Design review of the part built by this model. Coordinates are the model's own, in mm. A direction names the side the tool comes from. Coordinates: 2 decimals unless noted, no trailing zeros. Write each loop counter-clockwise with the first axis right and the second up, starting at its lowest first coordinate (ties: lowest second). Pieces come first, ordered by that corner, then holes. Notation, with made-up numbers: (61, 10) - (119, 10) arc R13 ccw to (119, 26) - close; hole circle Ø2 at (5.25, 66). An arc over 180 degrees is marked (long way). Answer as a JSON object with one key per item and string values.
```python
from build123d import *

# Parameters (mm, degrees)
SKETCH1_R           = 19.05
BOSS_EXTRUDE1_DEPTH = 31.75
SKETCH3_R           = 6.35
CUT_EXTRUDE1_DEPTH  = 127.593613969


with BuildPart() as part:
    # Sketch1 → Boss-Extrude1 (new, symmetric)
    with BuildSketch(Plane.XY):
        with BuildLine():
            Line((-51.074053478, -18.968891898), (-51.074053478, -6.268891898))
            ThreePointArc((-51.074053478, -6.268891898), (-54.793797356, 2.711364223), (-63.774053478, 6.431108102))
            Line((-63.774053478, 6.431108102), (-106.700053478, 6.431108102))
            Line((-106.700053478, 6.431108102), (-106.700053478, 14.381308102))
            Line((-106.700053478, 14.381308102), (58.399946522, 14.381308102))
            Line((58.399946522, 14.381308102), (58.399946522, 6.431108102))
            Line((58.399946522, 6.431108102), (15.473946522, 6.431108102))
            ThreePointArc((15.473946522, 6.431108102), (6.493690401, 2.711364223), (2.773946522, -6.268891898))
            Line((2.773946522, -6.268891898), (2.773946522, -18.968891898))
            ThreePointArc((2.773946522, -18.968891898), (-24.150053478, -45.892891898), (-51.074053478, -18.968891898))
        make_face()
        with Locations((-24.150053478, -18.968891898)):
            Circle(SKETCH1_R, mode=Mode.SUBTRACT)
    extrude(amount=BOSS_EXTRUDE1_DEPTH, both=True)

    # Sketch3 → Cut-Extrude1 (cut, through all)
    with BuildSketch(Plane(origin=(0, 14.381308102, 0), x_dir=(1, 0, 0), z_dir=(0, 1, 0))):
        with Locations(Location((-87.650053478, 15.875, 0), (0, 0, 270))):
            Circle(SKETCH3_R)
        with Locations(Location((-87.650053478, -15.875, 0), (0, 0, 270))):
            Circle(SKETCH3_R)
        with Locations(Location((39.349946522, -15.875, 0), (0, 0, 270))):
            Circle(SKETCH3_R)
        with Locations(Location((39.349946522, 15.875, 0), (0, 0, 270))):
            Circle(SKETCH3_R)
    extrude(amount=-CUT_EXTRUDE1_DEPTH, mode=Mode.SUBTRACT)


solid = part.part
```
(1) The part is to be moulded in two halves that separate along X. For faces 4 (the face through (-85, 6.431, 0)), 5 (the face through (-5.98, -13.25, -0.44)), 6 (the face through (-23.558, -45.886, 0.444)), say which applies: pulls with the +X half, pulls with the -X half, needs draft (parallel to the pull), parting line crosses it, or undercut.
Solved:
{"face 4": "needs draft", "face 5": "undercut", "face 6": "parting line crosses it"}
(2) Tool access review of faces 1 (the face through (2.774, -13, 0)), 2 (the face through (-81.354, 10.462, -16.702)), 3 (the face through (-51.074, -13, 0)): name each direction out of +Z, -Z, +X, -X, +Y, -Y from which nothing blocks a thin tool from reaching the whole face with its end or side.
Solved:
{"face 1": "+Z, -Z, +X, -Y", "face 2": "+Y, -Y", "face 3": "+Z, -Z, -X, -Y"}
(3) Take a section at D-D, the plane z = 17. Write out the cut boundary in (x, y), and give its area (3 significant figures).
Solved:
{"outline": "(-106.7, 6.43) - (-93.9, 6.43) - (-93.9, 14.38) - (-106.7, 14.38) - close; (-81.4, 6.43) - (-63.77, 6.43) arc R12.7 cw to (-51.07, -6.27) - (-51.07, -18.97) arc R26.92 ccw to (2.77, -18.97) - (2.77, -6.27) arc R12.7 cw to (15.47, 6.43) - (33.1, 6.43) - (33.1, 14.38) - (-81.4, 14.38) - close; (45.6, 6.43) - (58.4, 6.43) - (58.4, 14.38) - (45.6, 14.38) - close; hole circle Ø38.1 at (-24.15, -18.97)", "area": "2,550 mm^2"}
(4) Take a section at B-B, the plane x = -39. Write out the cut boundary in (y, z), and give its area (3 significant figures).
Solved:
{"outline": "(-41.43, -31.75) - (-30.9, -31.75) - (-30.9, 31.75) - (-41.43, 31.75) - close; (-7.04, -31.75) - (14.38, -31.75) - (14.38, 31.75) - (-7.04, 31.75) - close", "area": "2,030 mm^2"}
(5) Take a section at C-C, the plane y = -26.5. Write out the cut boundary in (x, z).
Solved:
{"outline": "(-50, -31.75) - (-41.65, -31.75) - (-41.65, 31.75) - (-50, 31.75) - close; (-6.65, -31.75) - (1.7, -31.75) - (1.7, 31.75) - (-6.65, 31.75) - close"}
(6) Take a section at A-A, the plane z = -8. Write out the cut boundary in (x, y), and give its area (3 significant figures).
Solved:
{"outline": "(-106.7, 6.43) - (-63.77, 6.43) arc R12.7 cw to (-51.07, -6.27) - (-51.07, -18.97) arc R26.92 ccw to (2.77, -18.97) - (2.77, -6.27) arc R12.7 cw to (15.47, 6.43) - (58.4, 6.43) - (58.4, 14.38) - (-106.7, 14.38) - close; hole circle Ø38.1 at (-24.15, -18.97)", "area": "2,750 mm^2"}
(7) For pin 1 (14 mm diameter, centred on y = -9.5, z = 14.5, fed in from -X); pin 2 (20.5 mm diameter, centred on x = -87.65, z = 15.88, fed in from -Y); pin 3 (2 mm diameter, centred on y = 3.5, z = 2, fed in from +X), all flat-tipped, find the tip position at first contact; note any pin that passes through.
Solved:
{"pin 1": "stops at x = -51.65", "pin 2": "stops at y = 6.43", "pin 3": "stops at x = 8.74"}
(8) To check wall thickness, follow line 1 (X direction, y = 8, z = -15.5); line 2 (X direction, y = -19.5, z = 22.5); line 3 (Y direction, x = 50.5, z = -26.5). State the ranges of each line that lie inside material, in increasing order. Write a range as from..to.
Solved:
{"line 1": "x = -106.7..-93.99, -81.31..33.01, 45.69..58.4", "line 2": "x = -51.07..-43.19, -5.11..2.77", "line 3": "y = 6.43..14.38"}
